from build123d import *

# Parameters (mm, degrees)
SKETCH_1_W             = 316
SKETCH_1_H             = 244.9
EXTRUDE_1_DEPTH        = 6
CUT_EXTRUDE_START      = 6
SKETCH_1_3_W           = 316
SKETCH_1_3_H           = 244.9
SKETCH_1_3_W_2         = 304
SKETCH_1_3_H_2         = 232.9
CUT_EXTRUDE_1_DEPTH    = 1
HOLE_WIZARD_M3_1_D     = 3.2
HOLE_WIZARD_M3_2_D     = 3.2
PATTERN_LINEAR_1_COUNT = 11
PATTERN_LINEAR_1_PITCH = 30
PATTERN_LINEAR_2_COUNT = 8
PATTERN_LINEAR_2_PITCH = 30
CUT_EXTRUDE_2_DEPTH    = 2.5
SKETCH_6_R             = 2.6
SKETCH_6_R_2           = 1.6
SKETCH_6_R_3           = 5
CUT_EXTRUDE_3_DEPTH    = 200.985005688
M3X0_5_1_D             = 2.5
SKETCH_7_R             = 6
CUT_EXTRUDE_5_DEPTH    = 200.985005688


with BuildPart() as part:
    # ｽｹｯﾁ1 → ﾎﾞｽ - 押し出し1 (new body)
    with BuildSketch(Plane.XY):
        Rectangle(SKETCH_1_W, SKETCH_1_H)
    extrude(amount=EXTRUDE_1_DEPTH)

    # ｽｹｯﾁ1<3> → ｶｯﾄ - 押し出し1 (cut)
    with BuildSketch(Plane.XY.offset(CUT_EXTRUDE_START)):
        Rectangle(SKETCH_1_3_W, SKETCH_1_3_H)
        Rectangle(SKETCH_1_3_W_2, SKETCH_1_3_H_2, mode=Mode.SUBTRACT)
    extrude(amount=-CUT_EXTRUDE_1_DEPTH, mode=Mode.SUBTRACT)

    # M3 すきま穴1 (through all)
    with Locations(Plane(origin=(155, 105, 0), x_dir=(-1, 0, 0), z_dir=(0, 0, -1))):
        with Locations((0, 0), (310, 0)):
            hole_wizard_m3_1 = Hole(HOLE_WIZARD_M3_1_D / 2)

    # M3 すきま穴2 (through all)
    with Locations(Plane(origin=(-150, 119.45, 0), x_dir=(-1, 0, 0), z_dir=(0, 0, -1))):
        with Locations((0, 0), (0, -238.9)):
            hole_wizard_m3_2 = Hole(HOLE_WIZARD_M3_2_D / 2)

    # 直線ﾊﾟﾀｰﾝ1: M3 すきま穴2 ×11
    with Locations(*[(i * PATTERN_LINEAR_1_PITCH, 0, 0) for i in range(1, PATTERN_LINEAR_1_COUNT)]):
        add(hole_wizard_m3_2, mode=Mode.SUBTRACT)

    # 直線ﾊﾟﾀｰﾝ2: M3 すきま穴1 ×8
    with Locations(*[(0, -i * PATTERN_LINEAR_2_PITCH, 0) for i in range(1, PATTERN_LINEAR_2_COUNT)]):
        add(hole_wizard_m3_1, mode=Mode.SUBTRACT)

    # ｽｹｯﾁ5 → ｶｯﾄ - 押し出し2 (cut)
    with BuildSketch(Plane.XY.offset(6)):
        Polygon((-3, -6.054864529), (-3, -113.45), (-144.047820055, -113.45), align=None)
        Polygon((-149, 109.679363659), (-8.892241646, 3), (-149, 3), align=None)
        Polygon((144.047820055, 113.45), (3, 113.45), (3, 6.054864529), align=None)
        Polygon((149, -109.679363659), (149, -3), (8.892241646, -3), align=None)
        Polygon((-144.047820055, 113.45), (-3, 6.054864529), (-3, 113.45), align=None)
        Polygon((3, -6.054864529), (144.047820055, -113.45), (3, -113.45), align=None)
        Polygon((-149, -109.679363659), (-8.892241646, -3), (-149, -3), align=None)
        Polygon((149, 3), (149, 109.679363659), (8.892241646, 3), align=None)
    extrude(amount=-CUT_EXTRUDE_2_DEPTH, mode=Mode.SUBTRACT)

    # ｽｹｯﾁ6 → ｶｯﾄ - 押し出し3 (cut, through all)
    with BuildSketch(Plane.XY.offset(6)):
        with Locations((10, -24)):
            Circle(SKETCH_6_R)
        with Locations((10, 50)):
            Circle(SKETCH_6_R)
        with Locations((10, -98.8)):
            Circle(SKETCH_6_R_2)
        with Locations((-6.281277591, -70.6)):
            Circle(SKETCH_6_R_2)
        with Locations((26.281277591, -70.6)):
            Circle(SKETCH_6_R_2)
        with Locations((10, -80)):
            Circle(SKETCH_6_R_3)
    extrude(amount=-CUT_EXTRUDE_3_DEPTH, mode=Mode.SUBTRACT)

    # M3x0.5 ねじ穴1 (through all)
    with Locations(Plane(origin=(0, 0, 0), x_dir=(-1, 0, 0), z_dir=(0, 0, -1))):
        with Locations((-37.5, 84.45), (37.5, 84.45), (53.5, -19), (53.5, 19), (26.5, 19), (26.5, -19), (37.5, -84.45), (-37.5, -84.45)):
            Hole(M3X0_5_1_D / 2)

    # ｽｹｯﾁ7 → ｶｯﾄ - 押し出し5 (cut, through all)
    with BuildSketch(Plane(origin=(0, 0, 0), x_dir=(-1, 0, 0), z_dir=(0, 0, -1))):
        with Locations((40, 12.5)):
            Circle(SKETCH_7_R)
        with Locations(Location((40, -12.5, 0), (0, 0, 180))):
            Circle(SKETCH_7_R)
    extrude(amount=-CUT_EXTRUDE_5_DEPTH, mode=Mode.SUBTRACT)


solid = part.part
Can you work these out from the model? Positions are in its coordinate system, mm. A direction names the side the tool comes from. Round coordinates to 2 decimals unless told otherwise and drop trailing zeros. Loops run counter-clockwise (first coordinate to the right, second up) from the corner with the lowest first, then second, coordinate; pieces in that order, holes last. Notation, with made-up numbers: (65.25, 76) - (105.25, 76) arc R20 cw to (105.25, 88) - close; hole circle Ø3 at (11.25, 27). An arc over 180 degrees is marked (long way). Write item = value, one per line. Start each with the question number.
(1) If we section it at B-B (x = 113): Please give me the cut outline in (y, z).
(2) For faces 3 (the face through (-35.24, 8.85, 1.73)), 4 (the face through (-79.93, 57.09, 4.77)), which set-ups out of +Z, -Z, +X, -X, +Y, -Y let a thin tool reach every point of the face, with its end or its side?
(3) If we mould it in two halves opening along Y, with no side actions, what happens to faces 1 (the face through (-153, 1, 5)), 2 (the face through (109, 33, 3.5))? For each: released by +Y, released by -Y, zero draft, split by the parting line, or undercut.
(4) For P1, Ø3.5, axis at x = 155, y = -15, coming from the +Z side; P2, Ø0.5, axis at x = -68.5, z = 5.5, coming from the +Y side; P3, Ø8, axis at x = 15, y = -53.5, coming from the +Z side, each with a flat end and sliding along its axis, tell me the tip position at first contact or that it passes through.
(5) If I drill on probe 1 along Y at (x, z) = (37.5, 1.45); probe 2 along Y at (x, z) = (-53.5, 2.45); probe 3 along Y at (x, z) = (124.5, 4.7), over which ranges is the centre line in solid material (lowest first)? Write a range as [from, to].
(6) If we section it at A-A (y = -80): Please give me the cut outline in (x, z).
Ans:
q1.outline = (-122.45, 0) - (122.45, 0) - (122.45, 5) - (116.45, 5) - (116.45, 6) - (113.45, 6) - (113.45, 3.5) - (89.81, 3.5) - (89.81, 6) - (82.27, 6) - (82.27, 3.5) - (3, 3.5) - (3, 6) - (-3, 6) - (-3, 3.5) - (-82.27, 3.5) - (-82.27, 6) - (-89.81, 6) - (-89.81, 3.5) - (-113.45, 3.5) - (-113.45, 6) - (-116.45, 6) - (-116.45, 5) - (-122.45, 5) - close
q2.face_3 = +Z, -Z
q2.face_4 = +Z
q3.face_1 = zero draft
q3.face_2 = undercut
q4.P1 = 5
q4.P2 = 116.45
q4.P3 = 3.5
q5.probe_1 = [-122.45, -85.7], [-83.2, 83.2], [85.7, 122.45]
q5.probe_2 = [-122.45, -20.25], [-17.75, 17.75], [20.25, 122.45]
q5.probe_3 = [-122.45, -113.45], [-98.57, -91.02], [-3, 3], [91.02, 98.57], [113.45, 122.45]
q6.outline = (-158, 0) - (5, 0) - (5, 3.5) - (3, 3.5) - (3, 6) - (-3, 6) - (-3, 3.5) - (-100.12, 3.5) - (-100.12, 6) - (-110.02, 6) - (-110.02, 3.5) - (-149, 3.5) - (-149, 6) - (-152, 6) - (-152, 5) - (-158, 5) - close; (15, 0) - (158, 0) - (158, 5) - (152, 5) - (152, 6) - (149, 6) - (149, 3.5) - (110.02, 3.5) - (110.02, 6) - (100.12, 6) - (100.12, 3.5) - (15, 3.5) - close
